Here's how the part is built. I have some questions about the finished solid (model axes, mm). Face numbers are marked on the shaded views. A direction names the side the tool comes from. Round coordinates to 2 decimals unless told otherwise and drop trailing zeros. Order: outer loops, then holes, each group sorted by start corner. A loop starts at its lowest first (then second) coordinate and runs counter-clockwise, first axis right, second up. Notation, with made-up numbers: (-37.5, 62) - (3.5, 62) arc R28 cw to (3.5, 80) - close; hole circle Ø6 at (-14.75, -2.75). An arc over 180 degrees is marked (long way). Answer as a JSON object with one key per item and string values.
```python
from build123d import *

# Parameters (mm, degrees)
SKETCH1_R           = 4.6
SKETCH1_R_2         = 1.6
BOSS_EXTRUDE1_DEPTH = 3.499999985
SKETCH2_W           = 7
SKETCH2_H           = 3
BOSS_EXTRUDE2_DEPTH = 3.499999985
BOSS_EXTRUDE3_REACH = 19.457
FILLET5_R           = 1
SKETCH6_R           = 0.625
CUT_EXTRUDE1_DEPTH  = 20.935540653
FILLET1_R           = 0.2
BOSS_EXTRUDE4_DEPTH = 3.499999985
FILLET2_R           = 1
FILLET3_R           = 1
BOSS_EXTRUDE5_START = 3.5
SKETCH1_2_R         = 4.6
SKETCH1_2_R_2       = 1.6
BOSS_EXTRUDE5_DEPTH = 0.5
SKETCH9_OUTSIDE_W   = 29.857
SKETCH9_OUTSIDE_H   = 18.02
SKETCH9_OUTSIDE_R   = 2.4
CUT_EXTRUDE2_DEPTH  = 0.5
FILLET4_R           = 1


with BuildPart() as part:
    # Sketch1 → Boss-Extrude1 (new, symmetric)
    with BuildSketch(Plane.XY):
        Circle(SKETCH1_R)
        Circle(SKETCH1_R_2, mode=Mode.SUBTRACT)
    extrude(amount=BOSS_EXTRUDE1_DEPTH, both=True)

    # Sketch2 → Boss-Extrude2 (add, symmetric)
    with BuildSketch(Plane.XY):
        with BuildLine():
            Line((14.025, -6.1875), (5.025, -6.1875))
            ThreePointArc((5.025, -6.1875), (1.004374029, -5.567503073), (-2.642710133, -3.765113963))
            ThreePointArc((-2.642710133, -3.765113963), (2.053101866, -4.116402887), (4.597420853, -0.154017857))
            ThreePointArc((4.597420853, -0.154017857), (4.878013126, -0.882668274), (5.596860169, -1.1875))
            Line((5.596860169, -1.1875), (14.025, -1.1875))
            Line((14.025, -1.1875), (14.025, -6.1875))
        make_face()
        with Locations((9.525, -3.6875)):
            Rectangle(SKETCH2_W, SKETCH2_H, mode=Mode.SUBTRACT)
    extrude(amount=BOSS_EXTRUDE2_DEPTH, both=True)

    # Sketch3 → Boss-Extrude3 (add, up to next)
    with BuildSketch(Plane(origin=(0, -5.1875, 0), x_dir=(1, 0, 0), z_dir=(0, 1, 0)), mode=Mode.PRIVATE) as boss_extrude3_sk1:
        with BuildLine():
            Line((6.497484118, 0.369658741), (6.025, -3.499999985))
            Line((6.025, -3.499999985), (6.025, 3.499999985))
            Line((6.025, 3.499999985), (8.025, 3.499999985))
            Line((8.025, 3.499999985), (8.025, 2.655654345))
            ThreePointArc((8.025, 2.655654345), (6.989049687, 1.694537108), (6.497484118, 0.369658741))
        make_face()
    boss_extrude3_tool1 = extrude(boss_extrude3_sk1.sketch, amount=BOSS_EXTRUDE3_REACH, mode=Mode.PRIVATE) - part.part
    # Sketch3 → Boss-Extrude3 (add, up to next)
    with BuildSketch(Plane(origin=(0, -5.1875, 0), x_dir=(1, 0, 0), z_dir=(0, 1, 0)), mode=Mode.PRIVATE) as boss_extrude3_sk2:
        with BuildLine():
            Line((12.552515882, 0.369658741), (13.025, -3.499999985))
            Line((13.025, -3.499999985), (13.025, 3.499999985))
            Line((13.025, 3.499999985), (11.025, 3.499999985))
            Line((11.025, 3.499999985), (11.025, 2.655654345))
            ThreePointArc((11.025, 2.655654345), (12.060950313, 1.694537108), (12.552515882, 0.369658741))
        make_face()
    boss_extrude3_tool2 = extrude(boss_extrude3_sk2.sketch, amount=BOSS_EXTRUDE3_REACH, mode=Mode.PRIVATE) - part.part
    add(boss_extrude3_tool1.solids().sort_by_distance((6.671602, -5.1875, -1.728299))[0])
    add(boss_extrude3_tool2.solids().sort_by_distance((12.378398, -5.1875, -1.728299))[0])

    # Fillet5
    fillet5_edges = [part.edges().sort_by_distance(p)[0] for p in [
        (14.025, -6.1875, 0),
        (14.025, -1.1875, 0),
    ]]
    fillet(fillet5_edges, radius=FILLET5_R)

    # Sketch6 → Cut-Extrude1 (cut, through all)
    with BuildSketch(Plane(origin=(14.025, 0, 0), x_dir=(0, 0, -1), z_dir=(1, 0, 0))):
        with Locations((0, -6.1875)):
            Circle(SKETCH6_R)
    extrude(amount=-CUT_EXTRUDE1_DEPTH, mode=Mode.SUBTRACT)

    # Fillet1
    fillet1_edges = [part.edges().sort_by_distance(p)[0] for p in [
        (13.95202478, -5.562500075, 0.000306186),
        (9.025, -6.1875, -0.625),
        (0.988571933, -5.562500075, 0.000306187),
        (9.025, -6.1875, 0.625),
    ]]
    fillet(fillet1_edges, radius=FILLET1_R)

    # Sketch7 → Boss-Extrude4 (add, symmetric)
    with BuildSketch(Plane.XY):
        with BuildLine():
            Line((-4.6, -1), (-7.6, -1))
            ThreePointArc((-7.6, -1), (-8.6, 0), (-7.6, 1))
            Line((-7.6, 1), (-4.6, 1))
            ThreePointArc((-4.6, 1), (-3.6, 0), (-4.6, -1))
        make_face()
    extrude(amount=BOSS_EXTRUDE4_DEPTH, both=True)

    # Fillet2
    fillet2_edges = [part.edges().sort_by_distance(p)[0] for p in [
        (-4.491304348, 0.994075075, 0),
        (-4.491304348, -0.994075075, 0),
    ]]
    fillet(fillet2_edges, radius=FILLET2_R)

    # Fillet3
    fillet3_edges = [part.edges().sort_by_distance(p)[0] for p in [
        (11.025, -3.6875, -2.655654345),
        (8.025, -3.6875, -2.655654345),
    ]]
    fillet(fillet3_edges, radius=FILLET3_R)

    # Sketch1<2> → Boss-Extrude5 (add, symmetric)
    with BuildSketch(Plane.XY.offset(BOSS_EXTRUDE5_START)):
        with Locations(Location((0, 0, 0), (0, 0, 159.075167572))):
            Circle(SKETCH1_2_R)
        Circle(SKETCH1_2_R_2, mode=Mode.SUBTRACT)
    extrude(amount=BOSS_EXTRUDE5_DEPTH, both=True)

    # Sketch9 outside → Cut-Extrude2 (cut)
    with BuildSketch(Plane.XY.offset(3.999999985)):
        with Locations((2.7125, -0.794)):
            Rectangle(SKETCH9_OUTSIDE_W, SKETCH9_OUTSIDE_H)
        Circle(SKETCH9_OUTSIDE_R, mode=Mode.SUBTRACT)
    extrude(amount=-CUT_EXTRUDE2_DEPTH, mode=Mode.SUBTRACT)

    # Fillet4
    # the kernel refuses this fillet: 1 mm, written as the material it adds along each edge
    with BuildSketch(Plane(origin=(0, 0, 3.499999985), x_dir=(1, 0, 0), z_dir=(0, -1, 0))) as fillet4_piece_1:
        with BuildLine():
            CenterArc((3.266025404, 1), FILLET4_R, 210, 60)
            Line((2.4, 0.5), (2.382679492, 0.49))
            ThreePointArc((2.382679492, 0.49), (2.38, 0.25), (2.38, 0))
            Line((2.38, 0), (2.4, -0.02))
            Line((2.4, -0.02), (3.266025404, -0.02))
            Line((3.266025404, -0.02), (3.266025404, 0))
        make_face()
    revolve(axis=Axis((0, 0, 3.499999985), (0, 0, 1)))


solid = part.part
```
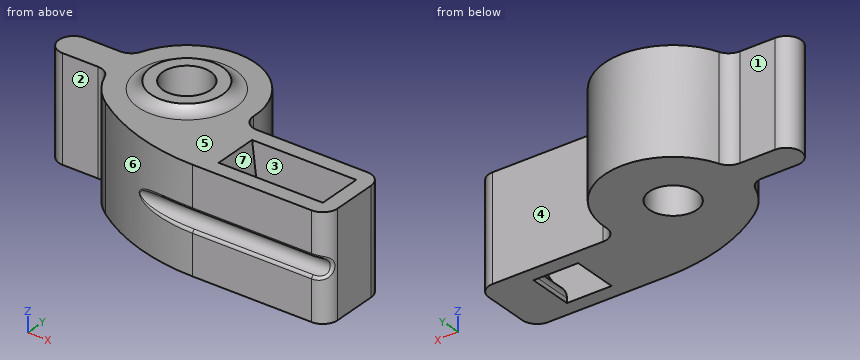
1. Imagine slicing it at B-B (x = 0). List the corners of the cut face in (y, z) for me.
Responses:
{"outline": "(-5.21, -3.5) - (-1.6, -3.5) - (-1.6, 4) - (-2.4, 4) arc R1 cw to (-3.27, 3.5) - (-5.21, 3.5) - close; (1.6, -3.5) - (4.6, -3.5) - (4.6, 3.5) - (3.27, 3.5) arc R1 cw to (2.4, 4) - (1.6, 4) - close"}
2. If I drill on L1, parallel to Y at x = 9.25, z = -1.25; L2, parallel to Z at x = -3, y = -3.25; L3, parallel to Y at x = 0, z = -1.5, over which ranges is the centre line in solid material (lowest first)? Write a range as [from, to].
Responses:
{"L1": "[-6.19, -5.19], [-2.19, -1.19]", "L2": "[-3.5, 3.5]", "L3": "[-5.21, -1.6], [1.6, 4.6]"}
3. Imagine slicing it at A-A (y = -3.5). List the corners of the cut face in (x, z) for me (3 decimals).
Responses:
{"outline": "(-2.985, -3.5) - (8.025, -3.5) - (8.025, -3.186) arc R1 ccw to (7.642, -2.4) arc R3.05 cw to (6.497, -0.37) - (6.025, 3.5) - (-2.985, 3.5) - close; (11.025, -3.5) - (14.025, -3.5) - (14.025, 3.5) - (13.025, 3.5) - (12.553, -0.37) arc R3.05 cw to (11.408, -2.4) arc R1 ccw to (11.025, -3.186) - close"}
4. Imagine slicing it at C-C (z = -2). Give the number of separate pieces and of enclosed holes in the cut face, plus the area to 3 significant figures.
Responses:
{"separate pieces": "1", "enclosed holes": "2", "area": "110 mm2"}
5. For P1, Ø2, axis at x = 9.5, z = 0.5, coming from the +Y side; P2, Ø2, axis at y = -5, z = 0, coming from the -X side; P3, Ø1.9, axis at x = -6, z = -1.5, coming from the +Y side, each with a flat end and sliding along its axis, tell me the tip position at first contact or that it passes through.
Responses:
{"P1": "y = -1.19", "P2": "x = -2.3", "P3": "y = 1.02"}
6. For the marked faces 1, 2, 3 and 4, which set-ups out of +Z, -Z, +X, -X, +Y, -Y let a thin tool reach every point of the face, with its end or its side?
Responses:
{"face 1": "+Z, -Z, -X, +Y", "face 2": "+Z, -Z, -X, -Y", "face 3": "+Z", "face 4": "+Z, -Z, +X, +Y"}
7. Thinking about a two-plate mould opening in X: for the marked faces 5, 6 and 7, which applies, pulls with the +X half, pulls with the -X half, needs draft (parallel to the pull), parting line crosses it, or undercut?
Responses:
{"face 5": "needs draft", "face 6": "pulls with the -X half", "face 7": "undercut"}
